Work out the finished part from the listing and answer in its coordinate system (mm). Face numbers are marked on the shaded views. A direction names the side the tool comes from. Coordinates: 2 decimals unless noted, no trailing zeros. Write each loop counter-clockwise with the first axis right and the second up, starting at its lowest first coordinate (ties: lowest second). Pieces come first, ordered by that corner, then holes. Notation, with made-up numbers: M 22,10 L 47,10 A25 ccw 47,46 Z; hole C -38.5,47 d9. An arc over 180 degrees is marked long. Answer as CSV lines item,"result". Start each with the question number.
(1) A cutting plane is placed at C-C on z = 0. Give the vertices of the cut face in (x, y), then the cut area to 3 significant figures.
(2) Flat-ended cylindrical pins translate along their axes: P1, Ø3, axis at y = -20, z = 0, coming from the -X side; P2, Ø2.5, axis at x = 0, z = 0, coming from the -Y side; P3, Ø4, axis at y = -17, z = -2.5, coming from the +X side. Find the tip coordinate at first contact, or state that the pin passes through.
(3) For the marked faces 1, 2 and 3, determine the directions among +Z, -Z, +X, -X, +Y, -Y from which every point of the face is accessible in a straight line to the end or side of a thin tool.
(4) A cutting plane is placed at B-B on x = 1.25. Give the vertices of the cut face in (y, z), then the cut area to 3 significant figures.
(5) Find the intervals of material crossed by L1, parallel to Y at x = -2.75, z = 2; L2, parallel to Y at x = -0.75, z = -1.75; L3, parallel to Z at x = 0, y = -20.95, in increasing order. Write a range as [from, to].
(6) The mould has two halves that part along X. Classify the marked faces 4 and 5: released by +X, released by -X, zero draft, split by the parting line, or undercut.
(7) A cutting plane is placed at D-D on x = -3.75. Give the vertices of the cut face in (y, z).
(8) A cutting plane is placed at A-A on y = -19.5. Give the vertices of the cut face in (x, z), then the cut area to 3 significant figures.
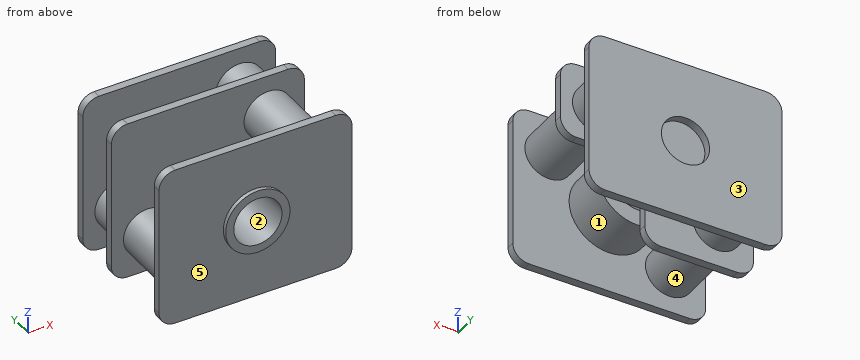
from build123d import *

# Parameters (mm, degrees)
SKETCH006_W     = 12
SKETCH006_H     = 10
PAD003_DEPTH    = 0.5
SKETCH007_R     = 1.5
PAD004_DEPTH    = 7.7
SKETCH008_W     = 12
SKETCH008_H     = 10
PAD005_DEPTH    = 0.5
SKETCH009_W     = 12
SKETCH009_H     = 10
PAD006_DEPTH    = 0.5
SKETCH010_R     = 2
PAD007_DEPTH    = 0.25
SKETCH011_R     = 2.5
PAD008_DEPTH    = 3
SKETCH012_R     = 1.5
POCKET003_DEPTH = 5
POCKET004_DEPTH = 1
FILLET_R        = 1
SKETCH014_R     = 1.5
POCKET005_DEPTH = 2


with BuildPart() as part:
    # Sketch006 (on DatumPlane) → Pad003 (new body)
    with BuildSketch(Plane.XZ.offset(14)):
        Rectangle(SKETCH006_W, SKETCH006_H)
    extrude(amount=PAD003_DEPTH)

    # Sketch007 (on Face6 of Pad003) → Pad004 (join)
    with BuildSketch(Plane.XZ.offset(14.5)):
        with Locations((3.75, 2.5)):
            Circle(SKETCH007_R)
        with Locations((-3.75, -2.5)):
            Circle(SKETCH007_R)
    extrude(amount=PAD004_DEPTH)

    # Sketch008 (on DatumPlane) → Pad005 (join)
    with BuildSketch(Plane.XZ.offset(17)):
        Rectangle(SKETCH008_W, SKETCH008_H)
    extrude(amount=PAD005_DEPTH)

    # Sketch009 (on DatumPlane) → Pad006 (join)
    with BuildSketch(Plane.XZ.offset(22)):
        Rectangle(SKETCH009_W, SKETCH009_H)
    extrude(amount=PAD006_DEPTH)

    # Sketch010 (on Face22 of Pad006) → Pad007 (join)
    with BuildSketch(Plane.XZ.offset(22.5)):
        Circle(SKETCH010_R)
    extrude(amount=PAD007_DEPTH)

    # Sketch011 (on Face17 of Pad007) → Pad008 (join)
    with BuildSketch(Plane(origin=(0, -22, 0), x_dir=(1, 0, 0), z_dir=(0, 1, 0))):
        Circle(SKETCH011_R)
    extrude(amount=PAD008_DEPTH)

    # Sketch012 (on Face26 of Pad008) → Pocket003 (cut)
    with BuildSketch(Plane.XZ.offset(22.75)):
        Circle(SKETCH012_R)
    extrude(amount=-POCKET003_DEPTH, mode=Mode.SUBTRACT)

    # Sketch013 (on Face14 of Pocket003) → Pocket004 (cut)
    with BuildSketch(Plane.XZ.offset(17.5)):
        with BuildLine():
            Line((7.000018, 0.25), (7.000018, -6))
            Line((7.000018, -6), (0.75, -6))
            Line((0.75, -2), (0.75, -6))
            ThreePointArc((3.000018, 0.25), (1.409016, -0.409003), (0.75, -2))
            Line((3.000018, 0.25), (7.000018, 0.25))
        make_face()
    extrude(amount=-POCKET004_DEPTH, mode=Mode.SUBTRACT)

    # Fillet
    fillet_edges = [part.edges().sort_by_distance(p)[0] for p in [
        (6, -22.25, 5),
        (6, -17.25, 5),
        (6, -14.25, 5),
        (-6, -22.25, 5),
        (-6, -17.25, 5),
        (-6, -14.25, 5),
        (-6, -22.25, -5),
        (-6, -17.25, -5),
        (-6, -14.25, -5),
        (6, -22.25, -5),
        (6, -14.25, -5),
        (6, -17.25, 0.25),
        (0.75, -17.25, -5),
    ]]
    fillet(fillet_edges, radius=FILLET_R)

    # Sketch014 (on Face2 of Fillet) → Pocket005 (cut)
    with BuildSketch(Plane(origin=(0, -14, 0), x_dir=(1, 0, 0), z_dir=(0, 1, 0))):
        Circle(SKETCH014_R)
    extrude(amount=-POCKET005_DEPTH, mode=Mode.SUBTRACT)


solid = part.part
Here are the results:
1,outline,"M -6,-22.5 L -2,-22.5 L -2,-22.75 L -1.5,-22.75 L -1.5,-19 L -2.5,-19 L -2.5,-22 L -6,-22 Z; M -6,-17.5 L 1.97,-17.5 L 1.97,-17 L -6,-17 Z; M -6,-14.5 L -1.5,-14.5 L -1.5,-14 L -6,-14 Z; M 1.5,-22.75 L 2,-22.75 L 2,-22.5 L 6,-22.5 L 6,-22 L 2.5,-22 L 2.5,-19 L 1.5,-19 Z; M 1.5,-14.5 L 6,-14.5 L 6,-14 L 1.5,-14 Z"
1,area,"19.2 mm^2"
2,P1,"stops at x = -4.87"
2,P2,"stops at y = -17.5"
2,P3,"stops at x = 1.32"
3,face 1,"none"
3,face 2,"-Y"
3,face 3,"+Z, -Z, +X, -X, +Y"
4,outline,"M -22.75,-1.56 L -22.5,-1.56 L -22.5,-5 L -22,-5 L -22,-2.17 L -19,-2.17 L -19,-0.83 L -22.75,-0.83 Z; M -22.75,0.83 L -19,0.83 L -19,2.17 L -22,2.17 L -22,5 L -22.5,5 L -22.5,1.56 L -22.75,1.56 Z; M -17.5,-0.59 L -17,-0.59 L -17,5 L -17.5,5 Z; M -14.5,-5 L -14,-5 L -14,-0.83 L -14.5,-0.83 Z; M -14.5,0.83 L -14,0.83 L -14,5 L -14.5,5 Z"
4,area,"19.5 mm^2"
5,L1,"y = [-22.5, -22], [-17.5, -17], [-14.5, -14]"
5,L2,"y = [-22.75, -19], [-17.5, -17], [-14.5, -14]"
5,L3,"z = [-2.5, -1.5], [1.5, 2.5]"
6,face 4,"undercut"
6,face 5,"zero draft"
7,outline,"M -22.5,-5 L -22,-5 L -22,-4 L -17.5,-4 L -17.5,-5 L -17,-5 L -17,-4 L -14.5,-4 L -14.5,-5 L -14,-5 L -14,5 L -14.5,5 L -14.5,-1 L -17,-1 L -17,5 L -17.5,5 L -17.5,-1 L -22,-1 L -22,5 L -22.5,5 Z"
8,outline,"C -3.75,-2.5 d3; C 0,0 d5; C 3.75,2.5 d3; hole C 0,0 d3"
8,area,"26.7 mm^2"
